from build123d import *

# Parameters (mm, degrees)
SKETCH1_W           = 19.05
SKETCH1_H           = 133.35
BOSS_EXTRUDE1_DEPTH = 584.2
SKETCH2_W           = 76.2
SKETCH2_H           = 19.05
SKETCH2_W_2         = 25.4
SKETCH2_H_2         = 28.575
CUT_EXTRUDE1_DEPTH  = 920.17672153
SKETCH3_W           = 6.35
SKETCH3_H           = 6.35
CUT_EXTRUDE2_DEPTH  = 49089.059018009


with BuildPart() as part:
    # Sketch1 → Boss-Extrude1 (new body)
    with BuildSketch(Plane.XY):
        with Locations((49069.931142185, 642.714387363)):
            Rectangle(SKETCH1_W, SKETCH1_H)
    extrude(amount=BOSS_EXTRUDE1_DEPTH)

    # Sketch2 → Cut-Extrude1 (cut, through all)
    with BuildSketch(Plane.ZY.offset(-49060.406142185)):
        with Locations((133.35, 642.714387363)):
            Rectangle(SKETCH2_W, SKETCH2_H)
        with Locations((450.85, 642.714387363)):
            Rectangle(SKETCH2_W, SKETCH2_H)
        with Locations((571.5, 695.101887363)):
            Rectangle(SKETCH2_W_2, SKETCH2_H_2)
        with Locations((12.7, 695.101887363)):
            Rectangle(SKETCH2_W_2, SKETCH2_H_2)
        with Locations((12.7, 590.326887363)):
            Rectangle(SKETCH2_W_2, SKETCH2_H_2)
        with Locations((571.5, 590.326887363)):
            Rectangle(SKETCH2_W_2, SKETCH2_H_2)
    extrude(amount=-CUT_EXTRUDE1_DEPTH, mode=Mode.SUBTRACT)

    # Sketch3 → Cut-Extrude2 (cut, through all)
    with BuildSketch(Plane.XY.offset(584.2)):
        with Locations((49063.581142185, 591.914387363)):
            Rectangle(SKETCH3_W, SKETCH3_H)
    extrude(amount=-CUT_EXTRUDE2_DEPTH, mode=Mode.SUBTRACT)


solid = part.part
Part model, mm, in its own coordinate system. A direction names the side the tool comes from. Coordinates: 2 decimals unless noted, no trailing zeros. Loops run counter-clockwise (first coordinate to the right, second up) from the corner with the lowest first, then second, coordinate; pieces in that order, holes last. Notation, with made-up numbers: (-5, -27.5) -> (12, -27.5) arc R30 cw to (12, -4.5) -> close; hole circle Ø6 at (-21, -15.5). An arc over 180 degrees is marked (long way). Use a Markdown table: item, result. Add a question column.
Item 1: Band-saw the part on D-D on y = 695.5. Write the cut outline in (x, z), plus the area to 3 significant figures.
Item 2: Pull direction Y, two halves, no side cores. Call faces 6 (the flat face through (49070, 643, 0)), 7 (the flat face through (49070, 709.389, 288)), 8 (the flat face through (49070, 633.189, 450)), 9 (the flat face through (49070, 643, 488.95)): +Y half, -Y half, draft (parallel to the pull), parting line (faces both ways), or undercut.
Item 3: Band-saw the part on C-C on x = 49070.5. Write the cut outline in (y, z), plus the area to 3 significant figures.
Item 4: Which spindle directions (+Z, -Z, +X, -X, +Y, -Y) get a long thin tool onto all of the face, cutting with end or side? Do faces 1 (the flat face through (49070, 680.814, 13)), 2 (the flat face through (49070, 604.614, 571)), 3 (the flat face through (49070, 643, 412.75)), 4 (the flat face through (49070, 604.614, 13)), 5 (the flat face through (49070, 680.814, 571)). Say none if no direction does.
Item 5: Flat gauge pins, fed straight in: P1, Ø1.9, axis at y = 592, z = 409.5, coming from the -X side; P2, Ø9.5, axis at x = 49065.5, y = 697, coming from the +Z side; P3, Ø5.5, axis at x = 49071, z = 9.5, coming from the +Y side. Where does each tip first touch, or does it go through?
Item 6: Band-saw the part on A-A on z = 431. Write the cut outline in (x, y).
Item 7: Probe probe 1 along Z at (x, y) = (49061.75, 646); probe 2 along Y at (x, z) = (49062.25, 250); probe 3 along Z at (x, y) = (49068.25, 585). List the from-to ranges inside material, lowest first.
Item 8: Band-saw the part on B-B on z = 517.5. Write the cut outline in (x, y).
Geometry says:
| question | item | result |
|---|---|---|
| 1 | outline | (49060.41, 25.4) -> (49079.46, 25.4) -> (49079.46, 558.8) -> (49060.41, 558.8) -> close |
| 1 | area | 10,200 mm² |
| 2 | face 6 | draft |
| 2 | face 7 | +Y half |
| 2 | face 8 | undercut |
| 2 | face 9 | undercut |
| 3 | outline | (576.04, 25.4) -> (604.61, 25.4) -> (604.61, 0) -> (680.81, 0) -> (680.81, 25.4) -> (709.39, 25.4) -> (709.39, 558.8) -> (680.81, 558.8) -> (680.81, 584.2) -> (604.61, 584.2) -> (604.61, 558.8) -> (576.04, 558.8) -> close; hole (633.19, 95.25) -> (652.24, 95.25) -> (652.24, 171.45) -> (633.19, 171.45) -> close; hole (633.19, 412.75) -> (652.24, 412.75) -> (652.24, 488.95) -> (633.19, 488.95) -> close |
| 3 | area | 72,100 mm² |
| 4 | face 1 | -Z, +X, -X, +Y |
| 4 | face 2 | +Z, +X, -X, -Y |
| 4 | face 3 | +X, -X |
| 4 | face 4 | -Z, +X, -X, -Y |
| 4 | face 5 | +Z, +X, -X, +Y |
| 5 | P1 | x = 49066.76 |
| 5 | P2 | z = 558.8 |
| 5 | P3 | y = 680.81 |
| 6 | outline | (49060.41, 576.04) -> (49079.46, 576.04) -> (49079.46, 633.19) -> (49060.41, 633.19) -> (49060.41, 595.09) -> (49066.76, 595.09) -> (49066.76, 588.74) -> (49060.41, 588.74) -> close; (49060.41, 652.24) -> (49079.46, 652.24) -> (49079.46, 709.39) -> (49060.41, 709.39) -> close |
| 7 | probe 1 | 0 to 95.25, 171.45 to 412.75, 488.95 to 584.2 |
| 7 | probe 2 | 576.04 to 588.74, 595.09 to 709.39 |
| 7 | probe 3 | 25.4 to 558.8 |
| 8 | outline | (49060.41, 576.04) -> (49079.46, 576.04) -> (49079.46, 709.39) -> (49060.41, 709.39) -> (49060.41, 595.09) -> (49066.76, 595.09) -> (49066.76, 588.74) -> (49060.41, 588.74) -> close |
